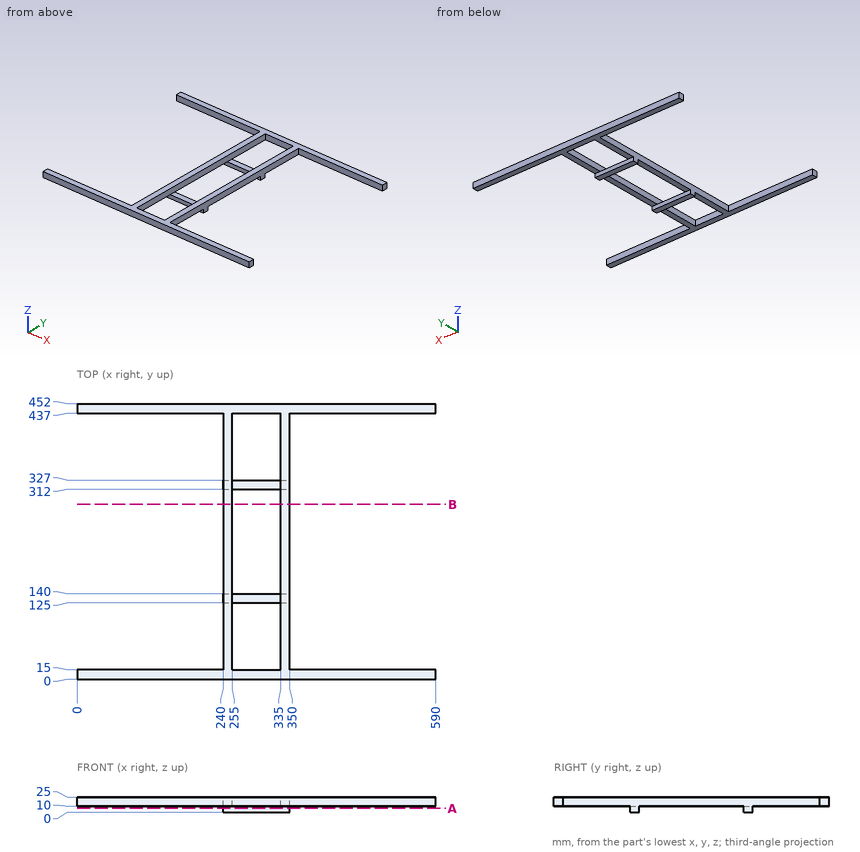
Can you work these out from the drawing? Everything is in mm from the part's minimum corner. Give positions to 0.01 mm unless a question says otherwise; leave off trailing zeros. Write each loop counter-clockwise with the first axis right and the second up, starting at its lowest first coordinate (ties: lowest second). Pieces come first, ordered by that corner, then holes. Notation, with made-up numbers: (72.25, -2) -> (117.25, -2) arc R22 cw to (117.25, 37) -> close; hole circle Ø3 at (81.25, 81). An arc over 180 degrees is marked (long way). Write each question's results on one line, items separated by ' | '. Start each with the question number.
Q1. I'm going to push flat-ended pins straight in: pin 1 Ø12 at (x, y) = (342.5, 194.5) entering from -Z; pin 2 Ø1.5 at (y, z) = (149, 13.5) entering from +X; pin 3 Ø3 at (y, z) = (256, 7.5) entering from -X; pin 4 Ø4.5 at (y, z) = (151, 21) entering from -X. Where does each tip first touch, or does it pass through?
Q2. I need wall thicknesses on probe 1 along Y at (x, z) = (150, 15.25); probe 2 along X at (y, z) = (291, 17); probe 3 along Y at (x, z) = (287, 4.25). Which ranges of each line are inside material? Lowest first, please.
Q3. Suppose I cut it at A-A, the plane z = 6.25. List the corners of the cut face in (x, y) for me, and give its area (3 significant figures).
Q4. Suppose I cut it at B-B, the plane y = 287. List the corners of the cut face in (x, z) for me, and give its area (3 significant figures).
Outcome:
1) pin 1: z = 10 | pin 2: x = 350 | pin 3: through | pin 4: x = 240
2) probe 1: 0 to 15, 437 to 452 | probe 2: 240 to 255, 335 to 350 | probe 3: 125 to 140, 312 to 327
3) outline: (240, 125) -> (350, 125) -> (350, 140) -> (240, 140) -> close; (240, 312) -> (350, 312) -> (350, 327) -> (240, 327) -> close | area: 3,300 mm2
4) outline: (240, 10) -> (255, 10) -> (255, 25) -> (240, 25) -> close; (335, 10) -> (350, 10) -> (350, 25) -> (335, 25) -> close | area: 450 mm2
